Part model, mm, in its own coordinate system. A direction names the side the tool comes from. Round coordinates to 2 decimals unless told otherwise and drop trailing zeros. Write each loop counter-clockwise with the first axis right and the second up, starting at its lowest first coordinate (ties: lowest second). Pieces come first, ordered by that corner, then holes. Notation, with made-up numbers: M 79,23 L 116,23 A16 cw 116,54 Z; hole C 14,61.5 d10. An arc over 180 degrees is marked long. Answer as a JSON object with one key per item and string values. Group by question number.
1. Band-saw the part on D-D, the plane y = 83. Write the cut outline in (x, z), plus the area to 3 significant figures.
2. Band-saw the part on A-A, the plane x = 0. Write the cut outline in (y, z).
3. Drill centre lines: line 1 (Y direction, x = 31, z = 3.5); line 2 (Y direction, x = 30.5, z = -49); line 3 (X direction, y = 43, z = 19.5). Where is each one in solid material? Low to high. Write a range as from..to.
4. Band-saw the part on C-C, the plane y = 16. Write the cut outline in (x, z).
5. Drop flat-ended pins along their axis: pin 1 (2 mm diameter, centred on y = 14.5, z = -21, fed in from -X); pin 2 (6 mm diameter, centred on x = -41, z = -3, fed in from +Y); pin 3 (1 mm diameter, centred on y = 46, z = -47.5, fed in from +X); pin 4 (6 mm diameter, centred on x = 46, z = -53, fed in from -Y). Give the stop position or say it passes through.
6. Which spindle directions (+Z, -Z, +X, -X, +Y, -Y) get a long thin tool onto all of the face, cutting with end or side? Do faces 1 (the face through (-61.99, 37.92, -13.77)), 2 (the face through (0, 63, -49.318)), 3 (the face through (-46.973, 63.322, 15.027)), 4 (the face through (46.973, 63.322, -15.027)). Say none if no direction does.
7. Band-saw the part on B-B, the plane z = 14. Write the cut outline in (x, y).
from build123d import *

# Parameters (mm, degrees)
SKETCH2_R           = 76.2
BOSS_EXTRUDE1_DEPTH = 25.4
SKETCH3_R           = 63.5
BOSS_EXTRUDE2_DEPTH = 25.4
BOSS_EXTRUDE3_DEPTH = 25.4
SKETCH5_R           = 3.81
BOSS_EXTRUDE4_DEPTH = 25.4


with BuildPart() as part:
    # Sketch2 → Boss-Extrude1 (new body)
    with BuildSketch(Plane(origin=(0, 0, 0), x_dir=(1, 0, 0), z_dir=(0, 1, 0))):
        with Locations(Location((0, 0, 0), (0, 0, 270))):
            Circle(SKETCH2_R)
    extrude(amount=BOSS_EXTRUDE1_DEPTH)

    # Sketch3 → Boss-Extrude2 (add)
    with BuildSketch(Plane(origin=(0, 25.4, 0), x_dir=(1, 0, 0), z_dir=(0, 1, 0))):
        with Locations(Location((0, 0, 0), (0, 0, 270))):
            Circle(SKETCH3_R)
    extrude(amount=BOSS_EXTRUDE2_DEPTH)

    # Sketch4 → Boss-Extrude3 (add)
    with BuildSketch(Plane(origin=(0, 50.8, 0), x_dir=(1, 0, 0), z_dir=(0, 1, 0))):
        Polygon((41.952120936, -30.48), (51.855673277, 0), (41.952120936, 30.48), (16.024284297, 49.317675977), (-16.024284297, 49.317675977), (-41.952120936, 30.48), (-51.855673277, 0), (-41.952120936, -30.48), (-16.024284297, -49.317675977), (16.024284297, -49.317675977), align=None)
    extrude(amount=BOSS_EXTRUDE3_DEPTH)

    # Sketch5 → Boss-Extrude4 (add)
    with BuildSketch(Plane(origin=(0, 76.2, 0), x_dir=(1, 0, 0), z_dir=(0, 1, 0))):
        with Locations(Location((12.7, 21.997045256, 0), (0, 0, 270))):
            Circle(SKETCH5_R)
    extrude(amount=BOSS_EXTRUDE4_DEPTH)


solid = part.part
Worked answers:
{
 "1": {"outline": "C 12.7,-22 d7.62", "area": "45.6 mm^2"},
 "2": {"outline": "M 0,-76.2 L 25.4,-76.2 L 25.4,-63.5 L 50.8,-63.5 L 50.8,-49.32 L 76.2,-49.32 L 76.2,49.32 L 50.8,49.32 L 50.8,63.5 L 25.4,63.5 L 25.4,76.2 L 0,76.2 Z"},
 "3": {"line 1": "y = 0..76.2", "line 2": "y = 0..50.8", "line 3": "x = -60.43..60.43"},
 "4": {"outline": "C 0,0 d152.4"},
 "5": {"pin 1": "stops at x = -73.53", "pin 2": "stops at y = 76.2", "pin 3": "stops at x = 42.7", "pin 4": "stops at y = 0"},
 "6": {"face 1": "+Y", "face 2": "-Z, +X, -X, +Y", "face 3": "+Z, -X, +Y", "face 4": "-Z, +X, +Y"},
 "7": {"outline": "M -74.9,0 L 74.9,0 L 74.9,25.4 L 61.94,25.4 L 61.94,50.8 L 47.31,50.8 L 47.31,76.2 L -47.31,76.2 L -47.31,50.8 L -61.94,50.8 L -61.94,25.4 L -74.9,25.4 Z"}
}
